Here's how the part is built. I have some questions about the finished solid (model axes, mm). Face numbers are marked on the shaded views. A direction names the side the tool comes from. Round coordinates to 2 decimals unless told otherwise and drop trailing zeros. Order: outer loops, then holes, each group sorted by start corner. A loop starts at its lowest first (then second) coordinate and runs counter-clockwise, first axis right, second up. Notation, with made-up numbers: (-13.75, -35.5) - (39.25, -35.5) arc R29 ccw to (39.25, -1.5) - close; hole circle Ø2 at (36, 86). An arc over 180 degrees is marked (long way). Answer as a JSON object with one key per item and string values.
```python
from build123d import *

# Parameters (mm, degrees)
SKETCH1_R           = 15
SKETCH1_R_2         = 0.9
BOSS_EXTRUDE1_DEPTH = 2
SKETCH1_3_R         = 4
SKETCH1_3_R_2       = 0.9
BOSS_EXTRUDE2_DEPTH = 30
BOSS_EXTRUDE3_DEPTH = 28
CHAMFER1_SIZE       = 28
CHAMFER1_SIZE_2     = 11


with BuildPart() as part:
    # Sketch1 → Boss-Extrude1 (new body)
    with BuildSketch(Plane.XY):
        Circle(SKETCH1_R)
        Circle(SKETCH1_R_2, mode=Mode.SUBTRACT)
    extrude(amount=BOSS_EXTRUDE1_DEPTH)

    # Sketch1<3> → Boss-Extrude2 (add)
    with BuildSketch(Plane.XY):
        Circle(SKETCH1_3_R)
        Circle(SKETCH1_3_R_2, mode=Mode.SUBTRACT)
    extrude(amount=BOSS_EXTRUDE2_DEPTH)

    # Sketch2 → Boss-Extrude3 (add)
    with BuildSketch(Plane.XY.offset(2)):
        with BuildLine():
            ThreePointArc((1.2, 14.951922953), (0, 15), (-1.2, 14.951922953))
            Line((-1.2, 14.951922953), (-1.2, 3.815756806))
            ThreePointArc((-1.2, 3.815756806), (0, 4), (1.2, 3.815756806))
            Line((1.2, 3.815756806), (1.2, 14.951922953))
        make_face()
        with BuildLine():
            Line((-3.815756806, 1.2), (-14.951922953, 1.2))
            ThreePointArc((-14.951922953, 1.2), (-15, 0), (-14.951922953, -1.2))
            Line((-14.951922953, -1.2), (-3.815756806, -1.2))
            ThreePointArc((-3.815756806, -1.2), (-4, 0), (-3.815756806, 1.2))
        make_face()
        with BuildLine():
            ThreePointArc((14.951922953, -1.2), (15, 0), (14.951922953, 1.2))
            Line((14.951922953, 1.2), (3.815756806, 1.2))
            ThreePointArc((3.815756806, 1.2), (4, 0), (3.815756806, -1.2))
            Line((3.815756806, -1.2), (14.951922953, -1.2))
        make_face()
        with BuildLine():
            Line((-1.2, -3.815756806), (-1.2, -14.951922953))
            ThreePointArc((-1.2, -14.951922953), (0, -15), (1.2, -14.951922953))
            Line((1.2, -14.951922953), (1.2, -3.815756806))
            ThreePointArc((1.2, -3.815756806), (0, -4), (-1.2, -3.815756806))
        make_face()
    extrude(amount=BOSS_EXTRUDE3_DEPTH)

    # Chamfer1
    # the kernel refuses this chamfer: 28, 11 mm, written as the material it takes off along each edge
    with BuildSketch(Plane(origin=(0, 0, 30), x_dir=(0.9999950652018581, 0.0031415874858912577, 0), z_dir=(0.0031415874858912577, -0.9999950652018581, 0))) as chamfer1_piece_1:
        Polygon((15, -CHAMFER1_SIZE), (15 - CHAMFER1_SIZE_2, 0), (15, 0), align=None)
    revolve(axis=Axis((0, 0, 30), (0, 0, 1)), revolution_arc=359.64, mode=Mode.SUBTRACT)
    with BuildSketch(Plane(origin=(0, 0, 30), x_dir=(0.0031415874858795345, -0.9999950652018582, 0), z_dir=(-0.9999950652018582, -0.0031415874858795345, 0))) as chamfer1_piece_2:
        Polygon((15, -CHAMFER1_SIZE), (15 - CHAMFER1_SIZE_2, 0), (15, 0), align=None)
    revolve(axis=Axis((0, 0, 30), (0, 0, 1)), revolution_arc=359.64, mode=Mode.SUBTRACT)
    with BuildSketch(Plane(origin=(0, 0, 30), x_dir=(-0.9999950652018582, -0.00314158748587628, 0), z_dir=(-0.00314158748587628, 0.9999950652018582, 0))) as chamfer1_piece_3:
        Polygon((15, -CHAMFER1_SIZE), (15 - CHAMFER1_SIZE_2, 0), (15, 0), align=None)
    revolve(axis=Axis((0, 0, 30), (0, 0, 1)), revolution_arc=359.64, mode=Mode.SUBTRACT)
    with BuildSketch(Plane(origin=(0, 0, 30), x_dir=(-0.003141587485897415, 0.9999950652018581, 0), z_dir=(0.9999950652018581, 0.003141587485897415, 0))) as chamfer1_piece_4:
        Polygon((15, -CHAMFER1_SIZE), (15 - CHAMFER1_SIZE_2, 0), (15, 0), align=None)
    revolve(axis=Axis((0, 0, 30), (0, 0, 1)), revolution_arc=359.64, mode=Mode.SUBTRACT)


solid = part.part
```
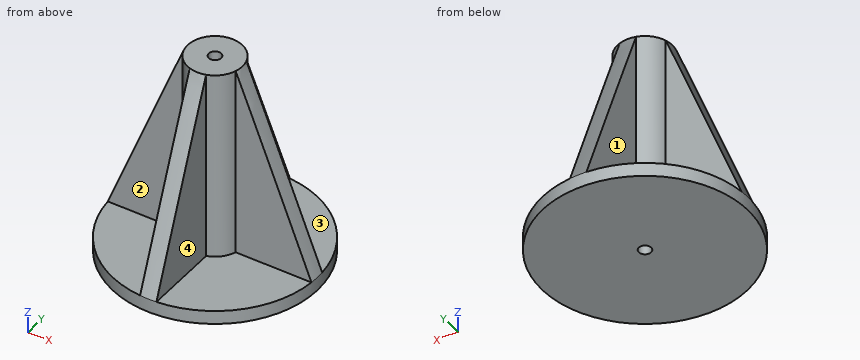
1. For the marked faces 1, 2, 3 and 4, which set-ups out of +Z, -Z, +X, -X, +Y, -Y let a thin tool reach every point of the face, with its end or its side?
Responses:
{"face 1": "+Z, -X, +Y", "face 2": "+Z, -X, -Y", "face 3": "+Z, +X, +Y", "face 4": "+Z, +X, -Y"}
2. For P1, Ø1, axis at y = 9.5, z = 9, coming from the -X side; P2, Ø12, axis at y = 11, z = 14, coming from the +X side; P3, Ø3, axis at y = -1, z = 27, coming from the +X side, each with a flat end and sliding along its axis, tell me the tip position at first contact or that it passes through.
Responses:
{"P1": "x = -1.2", "P2": "x = 1.2", "P3": "x = 5.72"}
3. Imagine slicing it at A-A (y = 0). List the corners of the cut face in (x, z) for me.
Responses:
{"outline": "(-15, 0) - (-0.9, 0) - (-0.9, 30) - (-4, 30) - (-15, 2) - close; (0.9, 0) - (15, 0) - (15, 2) - (4, 30) - (0.9, 30) - close"}
4. Imagine slicing it at C-C (z = 19.5). List the corners of the cut face in (x, y) for me (3 decimals), plus the area to 3 significant figures.
Responses:
{"outline": "(-8.036, -1.2) - (-3.816, -1.2) arc R4 ccw to (-1.2, -3.816) - (-1.2, -8.036) arc R8.125 ccw to (1.2, -8.036) - (1.2, -3.816) arc R4 ccw to (3.816, -1.2) - (8.036, -1.2) arc R8.125 ccw to (8.036, 1.2) - (3.816, 1.2) arc R4 ccw to (1.2, 3.816) - (1.2, 8.036) arc R8.125 ccw to (-1.2, 8.036) - (-1.2, 3.816) arc R4 ccw to (-3.816, 1.2) - (-8.036, 1.2) arc R8.125 ccw to start; hole circle Ø1.8 at (0, 0)", "area": "87.6 mm2"}
5. Imagine slicing it at D-D (y = -3). List the corners of the cut face in (x, z) for me, plus the area to 3 significant figures.
Responses:
{"outline": "(-14.7, 0) - (14.7, 0) - (14.7, 2) - (2.65, 2) - (2.65, 30) - (-2.65, 30) - (-2.65, 2) - (-14.7, 2) - close", "area": "207 mm2"}
6. If I drill on L1, parallel to Z at x = 7.5, y = -5.5; L2, parallel to X at y = 12.5, z = 8, over which ranges is the centre line in solid material (lowest first)? Write a range as [from, to].
Responses:
{"L1": "[0, 2]", "L2": "[-1.2, 1.2]"}
